For this review, take the finished solid that the model builds, in its own axes (mm). Face numbers are marked on the shaded views. A direction names the side the tool comes from. Coordinates: 2 decimals unless noted, no trailing zeros. Write each loop counter-clockwise with the first axis right and the second up, starting at its lowest first coordinate (ties: lowest second). Pieces come first, ordered by that corner, then holes. Notation, with made-up numbers: (46, -36) -> (50, -36) arc R26 ccw to (50, -21) -> close; hole circle Ø4 at (-20.5, -3.5). An arc over 180 degrees is marked (long way). Put each result on its own line as item: value. Start each with the question number.
Item 1: Insertion check: P1, Ø3, axis at x = -1.5, z = -6, coming from the +Y side; P2, Ø6, axis at y = 2.5, z = -7.5, coming from the +X side; P3, Ø6, axis at x = -4, z = -9, coming from the +Y side; P4, Ø1.8, axis at x = 21.2, y = 8, coming from the +Z side. Each pin has a flat end and moves straight along its axis. Give the tip position at first contact, or say it passes through.
Item 2: Consider section B-B on x = -21.2. Give the boundary of the cut face in (y, z), and give its area (3 significant figures).
Item 3: For the marked faces 3 and 4, list the 3-axis set-ups (+Z, -Z, +X, -X, +Y, -Y) from which the entire face can be reached by the end or side of a thin tool; tool diameter is ignored.
Item 4: Consider section A-A on z = 0.75. Give the number of separate pieces and of enclosed holes in the cut face, and give its area (3 significant figures).
Item 5: Consider section D-D on z = -6. Give the boundary of the cut face in (x, y).
Item 6: The part is to be moulded in two halves that separate along X. For the marked faces 1 and 2, say which applies: +X half, -X half, draft (parallel to the pull), parting line (faces both ways), or undercut.
Item 7: To check wall thickness, follow L1, parallel to Y at x = -11.3, z = 0.6; L2, parallel to Y at x = 21.2, z = 1.2; L3, parallel to Y at x = -3.81, z = 0.95. State the ranges of each line that lie inside material, in increasing order.
Item 8: Consider section C-C on x = 1.27. Give the boundary of the cut face in (y, z), and give its area (3 significant figures).
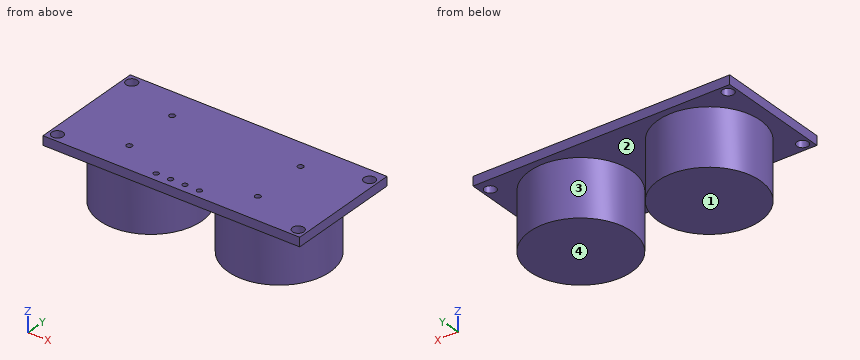
```python
from build123d import *

# Parameters (mm, degrees)
SKETCH_1_W          = 45.2
SKETCH_1_H          = 20.4
EXTRUDE_1_DEPTH     = 1.6
SKETCH_2_R          = 1
SKETCH_2_R_2        = 0.45
CUT_EXTRUDE_1_DEPTH = 25.846730167
SKETCH_3_R          = 0.5
CUT_EXTRUDE_2_DEPTH = 25.846730167
SKETCH_4_R          = 9
EXTRUDE_2_DEPTH     = 10


with BuildPart() as part:
    # Эскиз1 → Бобышка-Вытянуть1 (new body)
    with BuildSketch(Plane.XY):
        Rectangle(SKETCH_1_W, SKETCH_1_H)
    extrude(amount=EXTRUDE_1_DEPTH)

    # Эскиз2 → Вырез-Вытянуть1 (cut, through all)
    with BuildSketch(Plane.XY.offset(1.6)):
        with Locations((-21.2, 8.7)):
            Circle(SKETCH_2_R)
        with Locations((-21.2, -8.7)):
            Circle(SKETCH_2_R)
        with Locations((21.2, -8.7)):
            Circle(SKETCH_2_R)
        with Locations((21.2, 8)):
            Circle(SKETCH_2_R)
        with Locations((-3.81, -8.7)):
            Circle(SKETCH_2_R_2)
        with Locations((-1.27, -8.7)):
            Circle(SKETCH_2_R_2)
        with Locations((1.27, -8.7)):
            Circle(SKETCH_2_R_2)
        with Locations((3.81, -8.7)):
            Circle(SKETCH_2_R_2)
    extrude(amount=-CUT_EXTRUDE_1_DEPTH, mode=Mode.SUBTRACT)

    # Эскиз3 → Вырез-Вытянуть2 (cut, through all)
    with BuildSketch(Plane.XY.offset(1.6)):
        with Locations((11.3, 5)):
            Circle(SKETCH_3_R)
        with Locations((11.3, -5)):
            Circle(SKETCH_3_R)
        with Locations(Location((-11.3, -5, 0), (0, 0, 180))):
            Circle(SKETCH_3_R)
        with Locations(Location((-11.3, 5, 0), (0, 0, 180))):
            Circle(SKETCH_3_R)
    extrude(amount=-CUT_EXTRUDE_2_DEPTH, mode=Mode.SUBTRACT)

    # Эскиз4 → Бобышка-Вытянуть2 (add)
    with BuildSketch(Plane(origin=(0, 0, 0), x_dir=(-1, 0, 0), z_dir=(0, 0, -1))):
        with Locations(Location((-11.3, 0, 0), (0, 0, 180))):
            Circle(SKETCH_4_R)
        with Locations(Location((11.3, 0, 0), (0, 0, 180))):
            Circle(SKETCH_4_R)
    extrude(amount=EXTRUDE_2_DEPTH)


solid = part.part
```
Return value:
1. P1: y = 3.48
1. P2: x = 20.3
1. P3: y = 7.91
1. P4: through
2. outline: (-10.2, 0) -> (-9.7, 0) -> (-9.7, 1.6) -> (-10.2, 1.6) -> close; (-7.7, 0) -> (7.7, 0) -> (7.7, 1.6) -> (-7.7, 1.6) -> close; (9.7, 0) -> (10.2, 0) -> (10.2, 1.6) -> (9.7, 1.6) -> close
2. area: 26.2 mm^2
3. face 3: -Z
3. face 4: -Z, +X, -X, +Y, -Y
4. separate pieces: 1
4. enclosed holes: 12
4. area: 904 mm^2
5. outline: circle Ø18 at (-11.3, 0); circle Ø18 at (11.3, 0)
6. face 1: draft
6. face 2: undercut
7. L1: -10.2 to -5.5, -4.5 to 4.5, 5.5 to 10.2
7. L2: -10.2 to -9.7, -7.7 to 7, 9 to 10.2
7. L3: -10.2 to -9.15, -8.25 to 10.2
8. outline: (-10.2, 0) -> (-9.15, 0) -> (-9.15, 1.6) -> (-10.2, 1.6) -> close; (-8.25, 0) -> (10.2, 0) -> (10.2, 1.6) -> (-8.25, 1.6) -> close
8. area: 31.2 mm^2
